```python
from build123d import *

# Parameters (mm, degrees)
SKETCH_1_R          = 1
SKETCH_1_R_2        = 1.25
EXTRUDE_2_DEPTH     = 2
SKETCH_2_R          = 1.25
CUT_EXTRUDE_1_DEPTH = 10


with BuildPart() as part:
    # 草圖1 → 填料-伸長2 (new body)
    with BuildSketch(Plane.XY):
        with BuildLine():
            Line((55.038502783, 45.173220339), (55.038502783, 32.173220339))
            ThreePointArc((55.038502783, 32.173220339), (54.745609564, 31.466113558), (54.038502783, 31.173220339))
            Line((54.038502783, 31.173220339), (-90.763626261, 31.173220339))
            ThreePointArc((-90.763626261, 31.173220339), (-91.726620083, 31.171182694), (-92.665560041, 30.957283163))
            Line((-92.665560041, 30.957283163), (-92.665560041, 7.389157515))
            ThreePointArc((-92.665560041, 7.389157515), (-91.774171138, 6.395073197), (-90.689152782, 7.173220339))
            Line((-90.689152782, 7.173220339), (54.038502783, 7.173220339))
            ThreePointArc((54.038502783, 7.173220339), (54.745609564, 6.88032712), (55.038502783, 6.173220339))
            Line((55.038502783, 6.173220339), (55.038502783, -6.826779661))
            ThreePointArc((55.038502783, -6.826779661), (54.745609564, -7.533886442), (54.038502783, -7.826779661))
            Line((54.038502783, -7.826779661), (-91.881497217, -7.826779661))
            Line((-91.881497217, -7.826779661), (-91.881497217, -4.826779661))
            ThreePointArc((-91.881497217, -4.826779661), (-92.174390436, -4.11967288), (-92.881497217, -3.826779661))
            Line((-92.881497217, -3.826779661), (-94.881497217, -3.826779661))
            ThreePointArc((-94.881497217, -3.826779661), (-95.588603998, -4.11967288), (-95.881497217, -4.826779661))
            Line((-95.881497217, -4.826779661), (-95.881497217, -7.826779661))
            Line((-95.881497217, -7.826779661), (-97.881497217, -7.826779661))
            ThreePointArc((-97.881497217, -7.826779661), (-104.952565029, -4.897847473), (-107.881497217, 2.173220339))
            Line((-107.881497217, 2.173220339), (-107.881497217, 36.173220339))
            ThreePointArc((-107.881497217, 36.173220339), (-104.952565029, 43.244288151), (-97.881497217, 46.173220339))
            Line((-97.881497217, 46.173220339), (-95.881497217, 46.173220339))
            Line((-95.881497217, 46.173220339), (-95.881497217, 43.173220339))
            ThreePointArc((-95.881497217, 43.173220339), (-95.588603998, 42.466113558), (-94.881497217, 42.173220339))
            Line((-94.881497217, 42.173220339), (-92.881497217, 42.173220339))
            ThreePointArc((-92.881497217, 42.173220339), (-92.174390436, 42.466113558), (-91.881497217, 43.173220339))
            Line((-91.881497217, 43.173220339), (-91.881497217, 46.173220339))
            Line((-91.881497217, 46.173220339), (54.038502783, 46.173220339))
            ThreePointArc((54.038502783, 46.173220339), (54.745609564, 45.88032712), (55.038502783, 45.173220339))
        make_face()
        with Locations((-97.881497217, 41.173220339)):
            Circle(SKETCH_1_R, mode=Mode.SUBTRACT)
        with Locations((-89.881497217, 41.173220339)):
            Circle(SKETCH_1_R, mode=Mode.SUBTRACT)
        with Locations((-89.881497217, -2.826779661)):
            Circle(SKETCH_1_R, mode=Mode.SUBTRACT)
        with Locations((-97.881497217, -2.826779661)):
            Circle(SKETCH_1_R, mode=Mode.SUBTRACT)
        with Locations((50.038502783, 38.673220339)):
            Circle(SKETCH_1_R_2, mode=Mode.SUBTRACT)
        with Locations((50.038502783, -0.326779661)):
            Circle(SKETCH_1_R_2, mode=Mode.SUBTRACT)
        with BuildLine():
            Line((-74.961497217, -2.826779661), (-74.961497217, 2.173220339))
            ThreePointArc((-74.961497217, 2.173220339), (-73.961497217, 3.173220339), (-72.961497217, 2.173220339))
            Line((-72.961497217, 2.173220339), (43.038502783, 2.173220339))
            ThreePointArc((43.038502783, 2.173220339), (44.038502783, 3.173220339), (45.038502783, 2.173220339))
            Line((45.038502783, 2.173220339), (45.038502783, -2.826779661))
            ThreePointArc((45.038502783, -2.826779661), (44.038502783, -3.826779661), (43.038502783, -2.826779661))
            Line((43.038502783, -2.826779661), (-72.961497217, -2.826779661))
            ThreePointArc((-72.961497217, -2.826779661), (-73.961497217, -3.826779661), (-74.961497217, -2.826779661))
        make_face(mode=Mode.SUBTRACT)
        with BuildLine():
            Line((43.038502783, 41.173220339), (-72.961497217, 41.173220339))
            ThreePointArc((-72.961497217, 41.173220339), (-73.961497217, 42.173220339), (-74.961497217, 41.173220339))
            Line((-74.961497217, 41.173220339), (-74.961497217, 36.173220339))
            ThreePointArc((-74.961497217, 36.173220339), (-73.961497217, 35.173220339), (-72.961497217, 36.173220339))
            Line((-72.961497217, 36.173220339), (43.038502783, 36.173220339))
            ThreePointArc((43.038502783, 36.173220339), (44.038502783, 35.173220339), (45.038502783, 36.173220339))
            Line((45.038502783, 36.173220339), (45.038502783, 41.173220339))
            ThreePointArc((45.038502783, 41.173220339), (44.038502783, 42.173220339), (43.038502783, 41.173220339))
        make_face(mode=Mode.SUBTRACT)
    extrude(amount=EXTRUDE_2_DEPTH)

    # 草圖2 → 除料-伸長1 (cut)
    with BuildSketch(Plane.XY.offset(2)):
        with Locations((-77.461497217, -0.326779661)):
            Circle(SKETCH_2_R)
        with Locations((40.038502783, 4.673220339)):
            Circle(SKETCH_2_R)
        with Locations((40.038502783, -5.326779661)):
            Circle(SKETCH_2_R)
    extrude(amount=-CUT_EXTRUDE_1_DEPTH, mode=Mode.SUBTRACT)


solid = part.part
```
Could you check a few things on this model? Use its own coordinates, in mm. Give positions to 0.01 mm unless a question says otherwise; leave off trailing zeros. Loops run counter-clockwise (first coordinate to the right, second up) from the corner with the lowest first, then second, coordinate; pieces in that order, holes last. Notation, with made-up numbers: (-35, 38) - (-23, 38) arc R16 ccw to (-23, 47) - close; hole circle Ø9 at (27.25, -19). An arc over 180 degrees is marked (long way). Use one line per item in the form item = value.
1. I need wall thicknesses on probe 1 along Y at (x, z) = (-58, 1.55); probe 2 along X at (y, z) = (37, 0.2); probe 3 along Y at (x, z) = (-85, 1.55). Which ranges of each line are inside material? Lowest first, please.
Response values:
probe_1 = -7.83 to -2.83, 2.17 to 7.17, 31.17 to 36.17, 41.17 to 46.17
probe_2 = -107.85 to -74.96, 45.04 to 55.04
probe_3 = -7.83 to 7.17, 31.17 to 46.17
2. I'm going to push flat-ended pins straight in: pin 1 Ø0.6 at (x, z) = (-93.5, 0.5) entering from -Y; pin 2 Ø0.6 at (y, z) = (0.5, 1) entering from -X; pin 3 Ø0.6 at (y, z) = (38.5, 1) entering from -X. Where does each tip first touch, or does it pass through?
Response values:
pin_1 = -3.83
pin_2 = -107.79
pin_3 = -107.67
3. I want a section at A-A (x = 2.5). Please give me the cut outline in (y, z).
Response values:
outline = (-7.83, 0) - (-2.83, 0) - (-2.83, 2) - (-7.83, 2) - close; (2.17, 0) - (7.17, 0) - (7.17, 2) - (2.17, 2) - close; (31.17, 0) - (36.17, 0) - (36.17, 2) - (31.17, 2) - close; (41.17, 0) - (46.17, 0) - (46.17, 2) - (41.17, 2) - close
4. I want a section at B-B (y = 21). Please give me the cut outline in (x, z).
Response values:
outline = (-107.88, 0) - (-92.67, 0) - (-92.67, 2) - (-107.88, 2) - close
5. I want a section at C-C (z = 0.3). Give the number of separate pieces and of enclosed holes in the cut face, and give its area (3 significant figures).
Response values:
separate_pieces = 1
enclosed_holes = 11
area = 3,930 mm²
